For this review, take the finished solid that the model builds, in its own axes (mm). A direction names the side the tool comes from. Round coordinates to 2 decimals unless told otherwise and drop trailing zeros. Write each loop counter-clockwise with the first axis right and the second up, starting at its lowest first coordinate (ties: lowest second). Pieces come first, ordered by that corner, then holes. Notation, with made-up numbers: M -26,66 L 16,66 A8 ccw 16,72 Z; hole C 43,81 d9. An arc over 180 degrees is marked long. Use one line per item in the form item = value. Start each with the question number.
Item 1: Add section B-B (z = 513). State the section outline as (x, y) points, and give its area (3 significant figures).
Item 2: For faces 1 (the cylindrical face through (44.27, -295.14, 59.17)), 2 (the cylindrical face through (36.785, 326.818, 59.166)), 3 (the flat face through (-203.766, 12, 368)), list the 3-axis set-ups (+Z, -Z, +X, -X, +Y, -Y) from which the entire face can be reached by the end or side of a thin tool; tool diameter is ignored.
Item 3: Add section C-C (x = 125). State the section outline as (y, z) points, and give its area (3 significant figures).
Item 4: Add section A-A (y = 56). State the section outline as (x, z) points.
Item 5: For P1, Ø12, axis at y = -25.5, z = 608, coming from the +X side; P2, Ø10, axis at x = -0.5, y = -110.5, coming from the +Z side, all flat-tipped, find the tip position at first contact; note any pin that passes through.
Item 6: For line 1 (Z direction, x = 219.5, y = 288.5); line 2 (X direction, y = 22, z = 161), list the stretches that pass through material, from the lowest coordinate up. Write a range as [from, to].
from build123d import *

# Parameters (mm, degrees)
F0_W         = 503.2831068337
F0_H         = 635
F0_W_2       = 131.7168931663
F1_DEPTH     = 66.04
F2_W         = 100.6971086562
F2_H         = 635
F3_DEPTH     = 635
F4_R         = 22.86
F5_R         = 22.86
F6_R         = 22.86
F7_T1_DEPTH  = 100.33
F7_S5_W      = 22.86
F7_S5_H      = 22.86
F7_T6_DEPTH  = 22.86
F7_S11_W     = 22.86
F7_S11_H     = 22.86
F7_T12_DEPTH = 22.86


# Not quite as in the source:
# - a fillet or chamfer that OpenCascade refuses, or shapes differently, is made with other operations: its cross-section is extruded or revolved along the edge and cut away or added


with BuildPart() as f1:
    # F0 (on Top) → F1 (new body)
    with BuildSketch(Plane.XY):
        with Locations((-52.821796909, 15.8370759291)):
            Rectangle(F0_W, F0_H)
        with Locations((264.678203091, 15.8370759291)):
            Rectangle(F0_W_2, F0_H)
    extrude(amount=F1_DEPTH)

    # F2 (on face) → F3 (join)
    with BuildSketch(Plane.XY.offset(66.04)):
        with Locations((-254.1147959977, 15.8370759291)):
            Rectangle(F2_W, F2_H)
    extrude(amount=F3_DEPTH)

    # F4
    f4_edges = [f1.edges().sort_by_distance(p)[0] for p in [
        (-203.766242, 15.837076, 701.04),
        (-304.46335, 15.837076, 701.04),
    ]]
    fillet(f4_edges, radius=F4_R)

    # F5
    f5_edges = [f1.edges().sort_by_distance(p)[0] for p in [
        (-203.766242, -301.662924, 372.11),
        (63.385204, -301.662924, 66.04),
        (330.53665, 15.837076, 66.04),
        (63.385204, 333.337076, 66.04),
    ]]
    fillet(f5_edges, radius=F5_R)

    # F6
    f6_edges = [f1.edges().sort_by_distance(p)[0] for p in [
        (-203.766242, 333.337076, 372.11),
        (-304.46335, 333.337076, 339.09),
    ]]
    fillet(f6_edges, radius=F6_R)

    # F7: fillet of radius 22.86 on 2 edges, made by hand

    # F7_s2 → F7_t1 (cut)
    with BuildSketch(Plane.XY.offset(-57.15)):
        with BuildLine():
            ThreePointArc((307.6766496742, 333.3370759291), (323.8411106921, 326.641536947), (330.5366496742, 310.4770759291))
            Line((330.5366496742, 310.4770759291), (330.5366496742, 333.3370759291))
            Line((330.5366496742, 333.3370759291), (307.6766496742, 333.3370759291))
        make_face()
        with BuildLine():
            ThreePointArc((307.6766496742, -301.6629240709), (323.8411106921, -294.9673850888), (330.5366496742, -278.8029240709))
            Line((330.5366496742, -278.8029240709), (330.5366496742, -301.6629240709))
            Line((330.5366496742, -301.6629240709), (307.6766496742, -301.6629240709))
        make_face()
    extrude(amount=F7_T1_DEPTH, mode=Mode.SUBTRACT)


with BuildPart() as f7_tool4:
    # F7_s5 → F7_t6 (new body)
    with BuildSketch(Plane.XZ.offset(278.8029240709)):
        with Locations((319.1066496742, 54.61)):
            Rectangle(F7_S5_W, F7_S5_H)
    extrude(amount=F7_T6_DEPTH)

    # F7_s7 → F7_t8 (revolve, cut)
    with BuildSketch(Plane(origin=(307.6766496742, -278.8029240709, 43.18), x_dir=(-0.7071067812, 0, -0.7071067812), z_dir=(-0.7071067812, 0, 0.7071067812))):
        with BuildLine():
            ThreePointArc((0, -22.86), (22.86, 0), (0, 22.86))
            Line((0, 22.86), (0, -22.86))
        make_face()
    revolve(axis=Axis((307.6766496742, -278.8029240709, 43.18), (0, -1, 0)), mode=Mode.SUBTRACT)


with BuildPart() as f1_1:
    add(f1.part)

    # F7_t3: cut F7_tool4
    add(f7_tool4.part, mode=Mode.SUBTRACT)


with BuildPart() as f7_tool10:
    # F7_s11 → F7_t12 (new body)
    with BuildSketch(Plane.XZ.offset(-310.4770759291)):
        with Locations((319.1066496742, 54.61)):
            Rectangle(F7_S11_W, F7_S11_H)
    extrude(amount=-F7_T12_DEPTH)

    # F7_s13 → F7_t14 (revolve, cut)
    with BuildSketch(Plane(origin=(307.6766496742, 310.4770759291, 43.18), x_dir=(-0.7071067812, 0, -0.7071067812), z_dir=(0.7071067812, 0, -0.7071067812))):
        with BuildLine():
            ThreePointArc((0, -22.86), (22.86, 0), (0, 22.86))
            Line((0, 22.86), (0, -22.86))
        make_face()
    revolve(axis=Axis((307.6766496742, 310.4770759291, 43.18), (0, 1, 0)), mode=Mode.SUBTRACT)


with BuildPart() as f1_2:
    add(f1_1.part)

    # F7_t9: cut F7_tool10
    add(f7_tool10.part, mode=Mode.SUBTRACT)


solid = f1_2.part
Calculated:
q1.outline = M -304.46,-278.8 A22.86 ccw -281.6,-301.66 L -226.63,-301.66 A22.86 ccw -203.77,-278.8 L -203.77,310.48 A22.86 ccw -226.63,333.34 L -281.6,333.34 A22.86 ccw -304.46,310.48 Z
q1.area = 63,500 mm^2
q2.face_1 = +Z, +X, -Y
q2.face_2 = +Z, +X, +Y
q2.face_3 = +Z, +X, +Y, -Y
q3.outline = M -301.66,0 L 333.34,0 L 333.34,43.18 A22.86 ccw 310.48,66.04 L -278.8,66.04 A22.86 ccw -301.66,43.18 Z
q3.area = 41,700 mm^2
q4.outline = M -304.46,0 L 330.54,0 L 330.54,43.18 A22.86 ccw 307.68,66.04 L -203.77,66.04 L -203.77,678.18 A22.86 ccw -226.63,701.04 L -281.6,701.04 A22.86 ccw -304.46,678.18 Z
q5.P1 = -203.77
q5.P2 = 66.04
q6.line_1 = [0, 66.04]
q6.line_2 = [-304.46, -203.77]
